CAD build for the part. Positions are in the model's coordinates, mm. A direction names the side the tool comes from. Give positions to 0.01 mm unless a question says otherwise; leave off trailing zeros. Write each loop counter-clockwise with the first axis right and the second up, starting at its lowest first coordinate (ties: lowest second). Pieces come first, ordered by that corner, then holes. Notation, with made-up numbers: (37.5, 34.5) -> (49.5, 34.5) arc R23 cw to (49.5, 70.5) -> close; hole circle Ø7 at (22, 70.5). An arc over 180 degrees is marked (long way). Answer as a JSON object with one key per item and string values.
```python
from build123d import *

# Parameters (mm, degrees)
SKETCH_W        = 70
SKETCH_H        = 20
PAD_DEPTH       = 8.5
POCKET_DEPTH    = 20
PAD001_DEPTH    = 13
SKETCH003_R     = 1
POCKET001_DEPTH = 8
FILLET_R        = 1


with BuildPart() as part:
    # Sketch → Pad (new body)
    with BuildSketch(Plane.XY):
        with Locations((0, 10)):
            Rectangle(SKETCH_W, SKETCH_H)
    extrude(amount=PAD_DEPTH)

    # Sketch001 (on Face3 of Pad) → Pocket (cut)
    with BuildSketch(Plane.XZ):
        with BuildLine():
            Line((-22.5, 4), (22.5, 4))
            ThreePointArc((35, 0), (28.975662, 2.705192), (22.5, 4))
            Line((-35, 0), (35, 0))
            ThreePointArc((-22.5, 4), (-28.975662, 2.705192), (-35, 0))
        make_face()
    extrude(amount=-POCKET_DEPTH, mode=Mode.SUBTRACT)

    # Sketch002 (on Face6 of Pocket) → Pad001 (join)
    with BuildSketch(Plane.XY.offset(8.5)):
        Polygon((-5, 9), (-15, 9), (-15, 12), (-8, 12), (-8, 20), (-5, 20), align=None)
        Polygon((18.3, 9), (28.3, 9), (28.3, 12), (21.3, 12), (21.3, 20), (18.3, 20), align=None)
    extrude(amount=PAD001_DEPTH)

    # Sketch003 (on Face17 of Pad001) → Pocket001 (cut)
    with BuildSketch(Plane.XZ.offset(-9)):
        with Locations((-7.5, 15.25)):
            Circle(SKETCH003_R)
        with Locations((20.8, 15.25)):
            Circle(SKETCH003_R)
    extrude(amount=-POCKET001_DEPTH, mode=Mode.SUBTRACT)

    # Fillet
    fillet_edges = [part.edges().sort_by_distance(p)[0] for p in [
        (-21.5, 20, 8.5),
        (-35, 10, 8.5),
        (0, 0, 8.5),
        (35, 10, 8.5),
        (6.65, 20, 8.5),
        (28.15, 20, 8.5),
    ]]
    fillet(fillet_edges, radius=FILLET_R)


solid = part.part
```
1) Slice it at B-B (z = 15.25). List the corners of the cut face in (x, y).
Model answer:
{"outline": "(-15, 9) -> (-8.5, 9) -> (-8.5, 12) -> (-15, 12) -> close; (-8, 17) -> (-6.5, 17) -> (-6.5, 9) -> (-5, 9) -> (-5, 20) -> (-8, 20) -> close; (18.3, 9) -> (19.8, 9) -> (19.8, 17) -> (21.3, 17) -> (21.3, 20) -> (18.3, 20) -> close; (21.8, 9) -> (28.3, 9) -> (28.3, 12) -> (21.8, 12) -> close"}
2) Slice it at A-A (z = 20). List the corners of the cut face in (x, y).
Model answer:
{"outline": "(-15, 9) -> (-5, 9) -> (-5, 20) -> (-8, 20) -> (-8, 12) -> (-15, 12) -> close; (18.3, 9) -> (28.3, 9) -> (28.3, 12) -> (21.3, 12) -> (21.3, 20) -> (18.3, 20) -> close"}
3) Wall check: probe 1 along Z at (x, y) = (20.8, 11.75); probe 2 along X at (y, z) = (17.5, 17.75); probe 3 along Z at (x, y) = (3.5, 4.75). Give the ranges that are in metal, low to high.
Model answer:
{"probe 1": "z = 4 to 14.25, 16.25 to 21.5", "probe 2": "x = -8 to -5, 18.3 to 21.3", "probe 3": "z = 4 to 8.5"}
4) Mould opens along X. For faces 1 (the flat face through (-35, 10, 4)), 2 (the flat face through (21, 13, 21.5)), 3 (the flat face through (0, 10, 4)) say: released by +X, released by -X, zero draft, split by the parting line, or undercut.
Model answer:
{"face 1": "released by -X", "face 2": "zero draft", "face 3": "undercut"}
5) Pin check, flat tips, straight feed: pin 1 (9 mm diameter, centred on y = 17.5, z = 15.5, fed in from -X); pin 2 (1.5 mm diameter, centred on y = 10, z = 18, fed in from +X); pin 3 (2.5 mm diameter, centred on y = 10, z = 15.5, fed in from -X); pin 4 (6 mm diameter, centred on x = 10, z = 13, fed in from +Y). Stop position of each tip, or through.
Model answer:
{"pin 1": "stops at x = -8", "pin 2": "stops at x = 28.3", "pin 3": "stops at x = -15", "pin 4": "passes through"}
6) Slice it at D-D (y = 3.5). List the corners of the cut face in (x, z).
Model answer:
{"outline": "(-35, 0) arc R29.45 cw to (-22.5, 4) -> (22.5, 4) arc R29.45 cw to (35, 0) -> (35, 7.5) arc R1 ccw to (34, 8.5) -> (-34, 8.5) arc R1 ccw to (-35, 7.5) -> close"}
7) 3-axis set-ups, long thin cutter, end or side, ignore diameter. For faces 4 (the flat face through (23, 9, 15)), 5 (the flat face through (-8, 18, 16)), 6 (the flat face through (21, 17, 15)), 7 (the flat face through (25, 12, 15)), 8 (the cylindrical face through (29.06, 9.86, 2.68)): which of +Z, -Z, +X, -X, +Y, -Y reach the whole face in a straight line?
Model answer:
{"face 4": "+Z, +X, -X, -Y", "face 5": "+Z, -X, +Y", "face 6": "-Y", "face 7": "+Z, +X, +Y", "face 8": "-Z, +Y, -Y"}
8) Slice it at C-C (y = 11.25). List the corners of the cut face in (x, z), then the cut area to 3 significant figures.
Model answer:
{"outline": "(-35, 0) arc R29.45 cw to (-22.5, 4) -> (22.5, 4) arc R29.45 cw to (35, 0) -> (35, 7.5) arc R1 ccw to (34, 8.5) -> (28.3, 8.5) -> (28.3, 21.5) -> (18.3, 21.5) -> (18.3, 8.5) -> (-5, 8.5) -> (-5, 21.5) -> (-15, 21.5) -> (-15, 8.5) -> (-34, 8.5) arc R1 ccw to (-35, 7.5) -> close; hole circle Ø2 at (-7.5, 15.25); hole circle Ø2 at (20.8, 15.25)", "area": "605 mm2"}
